Geometry: see drawing. Coordinates: mm, zero at the bounding-box minimum. Give positions to 0.01 mm unless a question says otherwise; leave off trailing zeros. Order: outer loops, then holes, each group sorted by start corner. A loop starts at its lowest first (then second) coordinate and runs counter-clockwise, first axis right, second up. Notation, with made-up numbers: M -26.5,-27.5 L 7.5,-27.5 A6 ccw 7.5,-23.5 Z; hole C 75.25,-17 d5. An arc over 180 degrees is marked long. Answer as a JSON object with one key per item and string values. Group by question number.
1. Material intervals for L1, parallel to Y at x = 5, z = 4.5; L2, parallel to X at y = 1.8, z = 5.25; L3, parallel to Z at x = 7.75, y = 1.3, sorted ascending. Write a range as [from, to].
2. Pin query (flat end, axial travel): P1, Ø1.5, axis at y = 4.5, z = 8, coming from the -X side. Return the tip coordinate at first contact, or that it passes through.
3. Section query B-B (z = 3.5). Output: boundary loops of the cut face in (x, y).
4. Section query A-A (x = 6.25). Output: boundary loops of the cut face in (y, z), plus the area to 3 significant figures.
5. Section query C-C (y = 1.8). Output: boundary loops of the cut face in (x, z), plus the area to 3 significant figures.
6. Section query D-D (x = 7.25). Output: boundary loops of the cut face in (y, z).
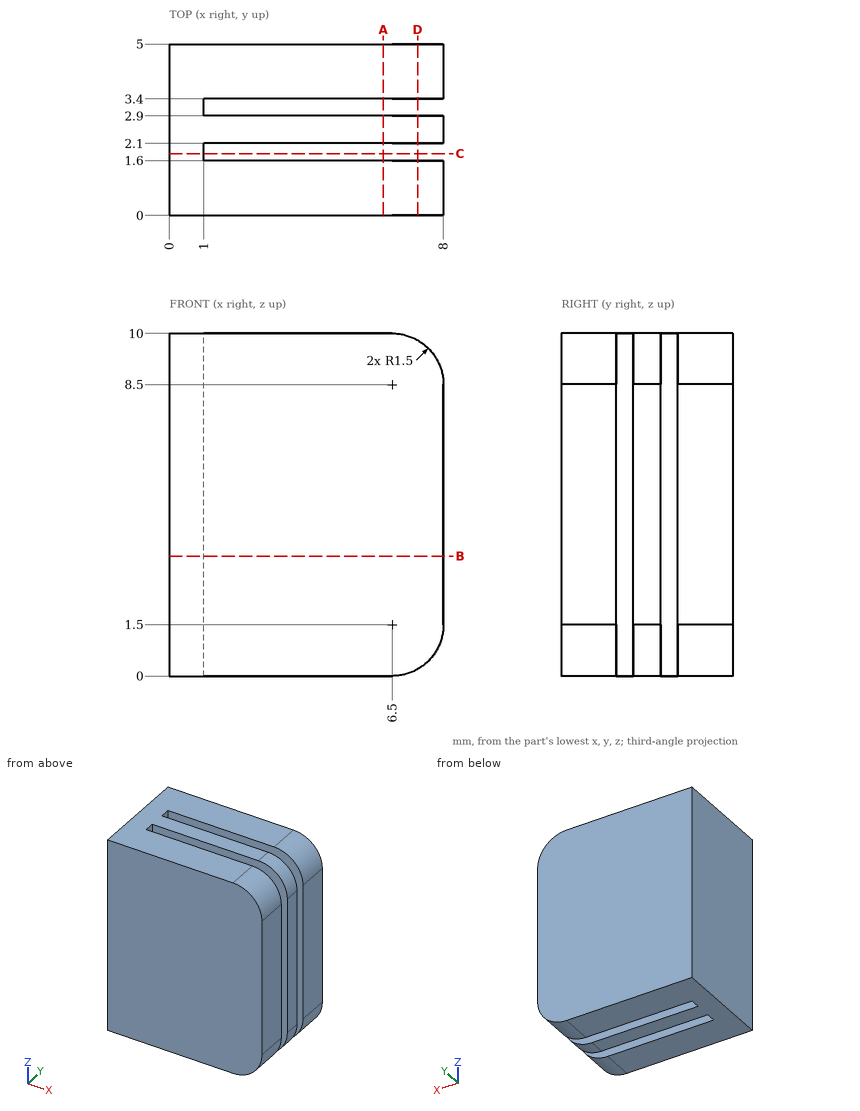
Answer sheet:
{
 "1": {"L1": "[0, 1.6], [2.1, 2.9], [3.4, 5]", "L2": "[0, 1]", "L3": "[0.67, 9.33]"},
 "2": {"P1": "x = 0"},
 "3": {"outline": "M 0,0 L 8,0 L 8,1.6 L 1,1.6 L 1,2.1 L 8,2.1 L 8,2.9 L 1,2.9 L 1,3.4 L 8,3.4 L 8,5 L 0,5 Z"},
 "4": {"outline": "M 0,0 L 1.6,0 L 1.6,10 L 0,10 Z; M 2.1,0 L 2.9,0 L 2.9,10 L 2.1,10 Z; M 3.4,0 L 5,0 L 5,10 L 3.4,10 Z", "area": "40.0 mm^2"},
 "5": {"outline": "M 0,0 L 1,0 L 1,10 L 0,10 Z", "area": "10.0 mm^2"},
 "6": {"outline": "M 0,0.2 L 1.6,0.2 L 1.6,9.8 L 0,9.8 Z; M 2.1,0.2 L 2.9,0.2 L 2.9,9.8 L 2.1,9.8 Z; M 3.4,0.2 L 5,0.2 L 5,9.8 L 3.4,9.8 Z"}
}
